Could you check a few things on this drawing? It's one solid part, dimensions in mm from its lowest x, y, z. A direction names the side the tool comes from. Round coordinates to 2 decimals unless told otherwise and drop trailing zeros. Write each loop counter-clockwise with the first axis right and the second up, starting at its lowest first coordinate (ties: lowest second). Pieces come first, ordered by that corner, then holes. Notation, with made-up numbers: (62.25, 77.25) -> (114.25, 77.25) arc R21 cw to (114.25, 101.25) -> close; hole circle Ø11 at (36, -16). An arc over 180 degrees is marked (long way). Answer in a Markdown table with one row per item.
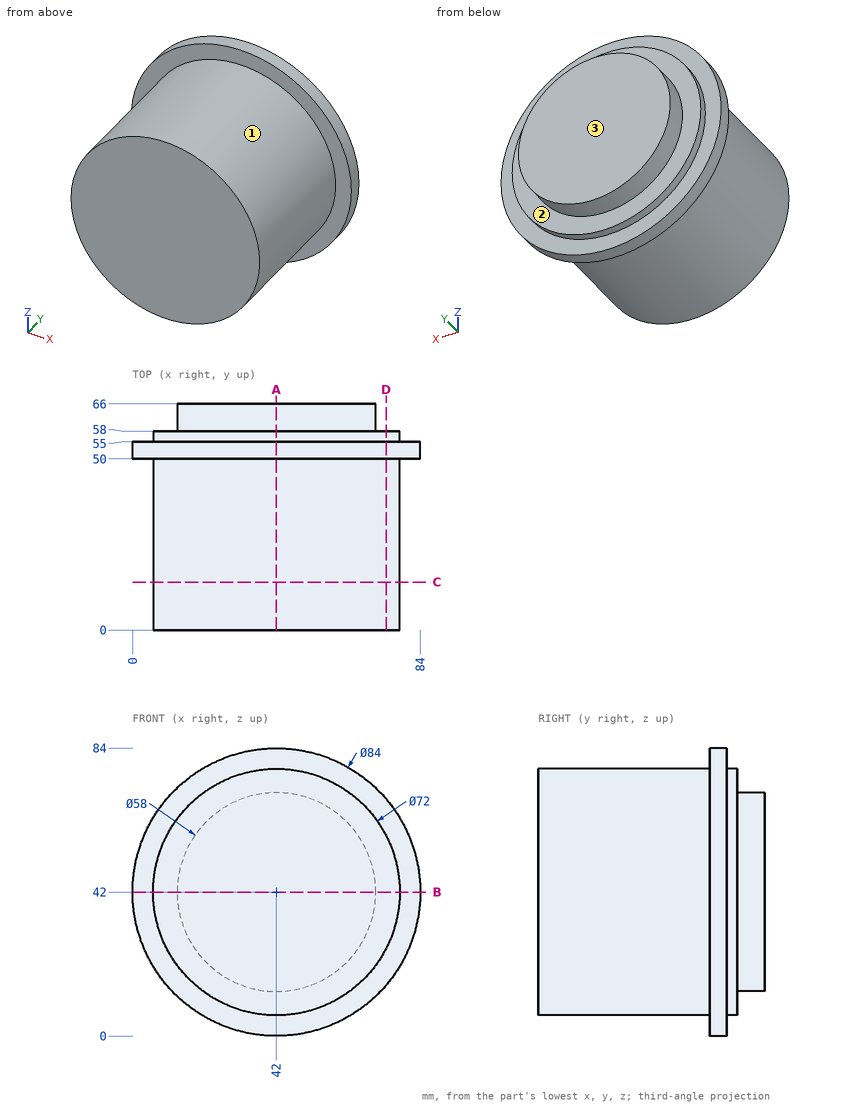
1) For pin 1 (12 mm diameter, centred on x = 20.5, y = 39, fed in from +Z); pin 2 (1 mm diameter, centred on y = 40, z = 30.5, fed in from +X); pin 3 (5 mm diameter, centred on x = 12.5, z = 14.5, fed in from -Y); pin 4 (12 mm diameter, centred on x = 10, z = 29.5, fed in from -Y), each with a flat end and sliding along its axis, tell me the tip position at first contact or that it passes through.
Findings:
| item | result |
|---|---|
| pin 1 | stops at z = 74.49 |
| pin 2 | stops at x = 76.28 |
| pin 3 | stops at y = 50 |
| pin 4 | stops at y = 0 |
2) For the marked faces 1, 2 and 3, which set-ups out of +Z, -Z, +X, -X, +Y, -Y let a thin tool reach every point of the face, with its end or its side?
Findings:
| item | result |
|---|---|
| face 1 | -Y |
| face 2 | +Y |
| face 3 | +Z, -Z, +X, -X, +Y |
3) Imagine slicing it at D-D, the plane x = 74. Please give me the cut outline in (y, z).
Findings:
| item | result |
|---|---|
| outline | (0, 25.51) -> (50, 25.51) -> (50, 14.8) -> (55, 14.8) -> (55, 25.51) -> (58, 25.51) -> (58, 58.49) -> (55, 58.49) -> (55, 69.2) -> (50, 69.2) -> (50, 58.49) -> (0, 58.49) -> close |
4) Imagine slicing it at C-C, the plane y = 14. Please give me the cut outline in (x, z).
Findings:
| item | result |
|---|---|
| outline | circle Ø72 at (42, 42) |
5) Please list where these lines run through material, in increasing order: line 1 (Y direction, x = 37, z = 77); line 2 (Y direction, x = 4.5, z = 48.5); line 3 (X direction, y = 37.5, z = 41.5).
Findings:
| item | result |
|---|---|
| line 1 | y = 0 to 58 |
| line 2 | y = 50 to 55 |
| line 3 | x = 6 to 78 |
6) Imagine slicing it at A-A, the plane x = 42. Please give me the cut outline in (y, z), plus the area to 3 significant figures.
Findings:
| item | result |
|---|---|
| outline | (0, 6) -> (50, 6) -> (50, 0) -> (55, 0) -> (55, 6) -> (58, 6) -> (58, 13) -> (66, 13) -> (66, 71) -> (58, 71) -> (58, 78) -> (55, 78) -> (55, 84) -> (50, 84) -> (50, 78) -> (0, 78) -> close |
| area | 4,700 mm^2 |
7) Imagine slicing it at B-B, the plane z = 42. Please give me the cut outline in (x, y), plus the area to 3 significant figures.
Findings:
| item | result |
|---|---|
| outline | (0, 50) -> (6, 50) -> (6, 0) -> (78, 0) -> (78, 50) -> (84, 50) -> (84, 55) -> (78, 55) -> (78, 58) -> (71, 58) -> (71, 66) -> (13, 66) -> (13, 58) -> (6, 58) -> (6, 55) -> (0, 55) -> close |
| area | 4,700 mm^2 |
